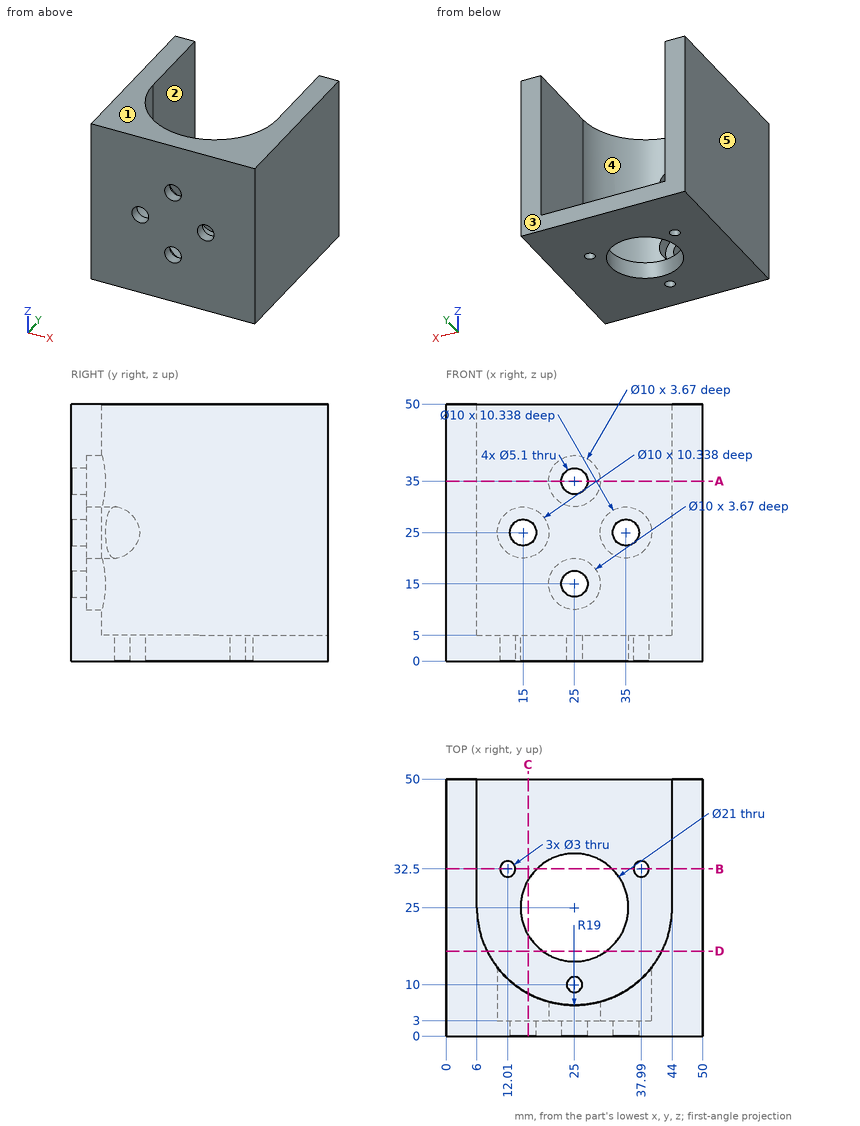
Design review of the part shown in the three views and the two pictorial views. Dimensions are in mm from the part's minimum x, y and z. A direction names the side the tool comes from. Coordinates: 2 decimals unless noted, no trailing zeros. Loops run counter-clockwise (first coordinate to the right, second up) from the corner with the lowest first, then second, coordinate; pieces in that order, holes last.
Q1. We need section B-B on y = 32.5. State the section outline as (x, z) points.
Reported:
outline: (0, 0) - (10.51, 0) - (10.51, 5) - (6, 5) - (6, 50) - (0, 50) - close; (13.51, 0) - (17.65, 0) - (17.65, 5) - (13.51, 5) - close; (32.35, 0) - (36.49, 0) - (36.49, 5) - (32.35, 5) - close; (39.49, 0) - (50, 0) - (50, 50) - (44, 50) - (44, 5) - (39.49, 5) - close
Q2. The part is to be moulded in two halves that separate along X. For the marked faces 3, 4 and 5, say which applies: +X half, -X half, draft (parallel to the pull), parting line (faces both ways), or undercut.
Reported:
face 3: draft
face 4: undercut
face 5: -X half
Q3. We need section C-C on x = 16. State the section outline as (y, z) points (1 decimal), and give its area (3 significant figures).
Reported:
outline: (0, 0) - (19.6, 0) - (19.6, 5) - (8.3, 5) - (8.3, 20.1) - (3, 20.1) - (3, 22.7) - (0, 22.7) - close; (0, 27.3) - (3, 27.3) - (3, 29.9) - (8.3, 29.9) - (8.3, 50) - (0, 50) - close; (30.4, 0) - (50, 0) - (50, 5) - (30.4, 5) - close
area: 502 mm2
Q4. We need section D-D on y = 16.5. State the section outline as (x, z) points (1 decimal).
Reported:
outline: (0, 0) - (18.8, 0) - (18.8, 5) - (8, 5) - (8, 50) - (0, 50) - close; (31.2, 0) - (50, 0) - (50, 50) - (42, 50) - (42, 5) - (31.2, 5) - close
Q5. To check wall thickness, follow line 1 (Z direction, x = 25, y = 1); line 2 (Z direction, x = 35, y = 8); line 3 (Z direction, x = 21, y = 4). State the ranges of each line that lie inside material, in increasing order.
Reported:
line 1: z = 0 to 12.45, 17.55 to 32.45, 37.55 to 50
line 2: z = 0 to 20, 30 to 50
line 3: z = 0 to 12, 18 to 32, 38 to 50
Q6. We need section A-A on z = 35. State the section outline as (x, y) points.
Reported:
outline: (0, 0) - (22.45, 0) - (22.45, 3) - (20, 3) - (20, 6.67) arc R19 cw to (6, 25) - (6, 50) - (0, 50) - close; (27.55, 0) - (50, 0) - (50, 50) - (44, 50) - (44, 25) arc R19 cw to (30, 6.67) - (30, 3) - (27.55, 3) - close
Q7. Tool access review of the marked faces 1 and 2: name each direction out of +Z, -Z, +X, -X, +Y, -Y from which nothing blocks a thin tool from reaching the whole face with its end or side.
Reported:
face 1: +Z, +X, -X, +Y, -Y
face 2: +Z, +Y
Q8. For pin 1 (6.5 mm diameter, centred on x = 15, z = 25, fed in from +Y); pin 2 (4.5 mm diameter, centred on x = 25, z = 15, fed in from -Y); pin 3 (4 mm diameter, centred on x = 25, y = 10, fed in from +Z); pin 4 (13 mm diameter, centred on x = 25, z = 15, fed in from +Y), all flat-tipped, find the tip position at first contact; note any pin that passes through.
Reported:
pin 1: stops at y = 3
pin 2: passes through
pin 3: stops at z = 5
pin 4: stops at y = 7.15
